Part model, mm, in its own coordinate system. A direction names the side the tool comes from. Give positions to 0.01 mm unless a question says otherwise; leave off trailing zeros. Order: outer loops, then holes, each group sorted by start corner. A loop starts at its lowest first (then second) coordinate and runs counter-clockwise, first axis right, second up. Notation, with made-up numbers: M 52,34 L 79,34 A28 cw 79,58 Z; hole C 53.25,-10 d4. An arc over 180 degrees is marked long. Return JSON: item names as keys, results as strings.
from build123d import *

# Parameters (mm, degrees)
SZKIC1_R                    = 15
DODANIE_WYCI_GNI_CIE1_DEPTH = 30
SZKIC2_R                    = 20
DODANIE_WYCI_GNI_CIE2_DEPTH = 2
DODANIE_WYCI_GNI_CIE3_START = -2
SZKIC3_R                    = 44
DODANIE_WYCI_GNI_CIE3_DEPTH = 15
DODANIE_WYCI_GNI_CIE4_START = -17
SZKIC4_R                    = 15
DODANIE_WYCI_GNI_CIE4_DEPTH = 10


with BuildPart() as part:
    # Szkic1 → Dodanie-wyciągnięcie1 (new body)
    with BuildSketch(Plane.XY):
        Circle(SZKIC1_R)
    extrude(amount=DODANIE_WYCI_GNI_CIE1_DEPTH)

    # Szkic2 → Dodanie-wyciągnięcie2 (add)
    with BuildSketch(Plane.XY):
        Circle(SZKIC2_R)
    extrude(amount=-DODANIE_WYCI_GNI_CIE2_DEPTH)

    # Szkic3 → Dodanie-wyciągnięcie3 (add)
    with BuildSketch(Plane.XY.offset(DODANIE_WYCI_GNI_CIE3_START)):
        Circle(SZKIC3_R)
    extrude(amount=-DODANIE_WYCI_GNI_CIE3_DEPTH)

    # Szkic4 → Dodanie-wyciągnięcie4 (add)
    with BuildSketch(Plane.XY.offset(DODANIE_WYCI_GNI_CIE4_START)):
        with Locations((0, 20)):
            Circle(SZKIC4_R)
    extrude(amount=-DODANIE_WYCI_GNI_CIE4_DEPTH)

    # Lustro2: part across plane


with BuildPart() as part_1:
    add(part.part)
    add(part.part.mirror(Plane(origin=(0, 20, -27), x_dir=(1, 0, 0), z_dir=(0, 0, 1))))


solid = part_1.part
Q1. Pin check, flat tips, straight feed: pin 1 (5 mm diameter, centred on x = 6, y = -33.5, fed in from +Z); pin 2 (5 mm diameter, centred on x = -11, z = -4, fed in from +Y); pin 3 (3 mm diameter, centred on y = 13.5, z = -30.5, fed in from +X). Stop position of each tip, or through.
Established:
{"pin 1": "stops at z = -2", "pin 2": "stops at y = 43.17", "pin 3": "stops at x = 14.14"}
Q2. Two-plate mould, pull along Z, no slides. Class faces 6 (the cylindrical face through (-9.538, -42.954, -9.395)), 7 (the flat face through (-1, 1, -37)), 8 (the flat face through (3, 15, -54)): +Z half, -Z half, draft (parallel to the pull), parting line (faces both ways), or undercut.
Established:
{"face 6": "draft", "face 7": "undercut", "face 8": "-Z half"}
Q3. Band-saw the part on A-A (y = 0). Give the cut face in (x, z), then the cut area to 3 significant figures.
Established:
{"outline": "M -44,-52 L -20,-52 L -20,-54 L -15,-54 L -15,-84 L 15,-84 L 15,-54 L 20,-54 L 20,-52 L 44,-52 L 44,-37 L -44,-37 Z; M -44,-17 L 44,-17 L 44,-2 L 20,-2 L 20,0 L 15,0 L 15,30 L -15,30 L -15,0 L -20,0 L -20,-2 L -44,-2 Z", "area": "4,600 mm²"}
Q4. Band-saw the part on D-D (z = -11). Give the cut face in (x, y), then the cut area to 3 significant figures.
Established:
{"outline": "C 0,0 d88", "area": "6,080 mm²"}
Q5. 3-axis set-ups, long thin cutter, end or side, ignore diameter. For faces 1 (the cylindrical face through (-14.985, 0.66, 14.79)), 2 (the cylindrical face through (-3.252, 5.357, -27.14)), 3 (the flat face through (0, 0, -84)), 4 (the cylindrical face through (-4.336, -19.524, -53.014)), 5 (the flat face through (0, 0, 30)): which of +Z, -Z, +X, -X, +Y, -Y reach the whole face in a straight line?
Established:
{"face 1": "+Z", "face 2": "none", "face 3": "-Z, +X, -X, +Y, -Y", "face 4": "-Z", "face 5": "+Z, +X, -X, +Y, -Y"}
Q6. Band-saw the part on C-C (x = -24). Give the cut face in (y, z).
Established:
{"outline": "M -36.88,-52 L 36.88,-52 L 36.88,-37 L -36.88,-37 Z; M -36.88,-17 L 36.88,-17 L 36.88,-2 L -36.88,-2 Z"}
Q7. Probe line 1 along Z through (x, y) = (-10, 1); line 2 along Z through (x, y) = (33.5, 20); line 3 along Y through (x, z) = (-0.5, -29). List the from-to ranges inside material, lowest first.
Established:
{"line 1": "z = -84 to -37, -17 to 30", "line 2": "z = -52 to -37, -17 to -2", "line 3": "y = 5.01 to 34.99"}
Q8. Band-saw the part on B-B (x = 0). Give the cut face in (y, z), then the cut area to 3 significant figures.
Established:
{"outline": "M -44,-52 L -20,-52 L -20,-54 L -15,-54 L -15,-84 L 15,-84 L 15,-54 L 20,-54 L 20,-52 L 44,-52 L 44,-37 L 35,-37 L 35,-17 L 44,-17 L 44,-2 L 20,-2 L 20,0 L 15,0 L 15,30 L -15,30 L -15,0 L -20,0 L -20,-2 L -44,-2 L -44,-17 L 5,-17 L 5,-37 L -44,-37 Z", "area": "5,200 mm²"}
